Verification items for the finished model (mm, model axes). Face numbers are marked on the shaded views. A direction names the side the tool comes from. Give positions to 0.01 mm unless a question says otherwise; leave off trailing zeros. Write each loop counter-clockwise with the first axis right and the second up, starting at its lowest first coordinate (ties: lowest second). Pieces come first, ordered by that corner, then holes. Notation, with made-up numbers: (-0.5, 11.5) - (9.5, 11.5) arc R35 ccw to (9.5, 44.5) - close; hole circle Ø6 at (-22, 51). An arc over 180 degrees is marked (long way). Put each result on its own line as item: value.
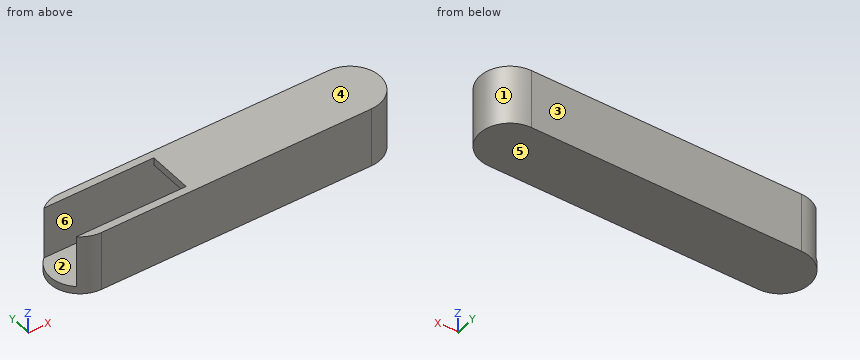
Autodesk Fusion 360 part; units mm, degrees
sketch "Sketch1" plane through (0, 0, 0) normal (0, 0, 1) x (1, 0, 0)
  line L0 (0, 0) -> (45, 0)
  line L1 (45, 10) -> (0, 10)
  arc A0 (0, 10) -> (0, 0) centre (0, 5) ccw
  arc A1 (45, 0) -> (45, 10) centre (45, 5) ccw
  dimension "d1" = 10
  dimension "d2" = 45
extrude "Extrude1" add sketch "Sketch1" along normal blind 10
sketch "Sketch2" plane through (0, 0, 0) normal (1, 0, 0) x (0, 1, 0)
  line L0 (1.25, 1.25) -> (8.75, 1.25)
  line L1 (8.75, 1.25) -> (8.75, 8.75)
  line L2 (8.75, 8.75) -> (1.25, 8.75)
  line L3 (1.25, 8.75) -> (1.25, 1.25)
  line L4 (10, 1.25) -> (8.75, 1.25) construction
  line L5 (0, 1.25) -> (1.25, 1.25) construction
  line L6 (0, 0) -> (0, 10)
  line L7 (10, 0) -> (10, 10)
  line L8 (8.75, 8.75) -> (8.75, 10) construction
  line L9 (8.75, 1.25) -> (8.75, 0) construction
  line L10 (10, 0) -> (0, 0)
  line L11 (10, 10) -> (0, 10)
  point P0 (10, 0)
  dimension "d5" = 7.5
  dimension "d6" = 7.5
extrude "Extrude2" cut sketch "Sketch2" along normal blind 45 and the other way through all contours L0 L1 L2 L3
sketch "Sketch3" plane through (0, 0, 10) normal (0, 0, 1) x (-1, 0, 0)
  arc A0 (-45, 0) -> (-45, -10) centre (-45, -5) ccw
  line L0 (-45, -10) -> (0, -10)
  arc A1 (0, -10) -> (0, 0) centre (0, -5) ccw
  line L1 (0, 0) -> (-45, 0)
  line L2 (5, -8.75) -> (-15, -8.75)
  line L3 (-15, -8.75) -> (-15, -1.25)
  line L4 (-15, -1.25) -> (5, -1.25)
  line L5 (5, -1.25) -> (5, -8.75)
  line L6 (5, -8.75) -> (5, -10) construction
  line L7 (5, -1.25) -> (5, 0) construction
  dimension "d11" = 7.5
  dimension "d12" = 30
extrude "Extrude3" cut sketch "Sketch3" against normal up to surface (1.25 mm away) contours A1 L2 L3 L4
Q1. Go/stop test with a flat-tipped pin: pin 1 Ø2 at (x, y) = (5.5, 4.5) entering from +Z. Record where the tip stops, or that it passes through.
Answers follow:
pin 1: stops at z = 1.25
Q2. Section check A-A, the plane x = 37.5. Record the cut outline in (y, z), plus the area to 4 significant figures.
Answers follow:
outline: (0, 0) - (10, 0) - (10, 10) - (0, 10) - close; hole (1.25, 1.25) - (8.75, 1.25) - (8.75, 8.75) - (1.25, 8.75) - close
area: 43.75 mm2
Q3. Section check C-C, the plane y = 5. Record the cut outline in (x, z), plus the area to 3 significant figures.
Answers follow:
outline: (-5, 0) - (50, 0) - (50, 10) - (15, 10) - (15, 8.75) - (45, 8.75) - (45, 1.25) - (-5, 1.25) - close
area: 150 mm2
Q4. Set-up check for the marked faces 5 and 6: record each of +Z, -Z, +X, -X, +Y, -Y from which the full face is reachable in a straight line by a thin tool's end or side.
Answers follow:
face 5: -Z, +X, -X, +Y, -Y
face 6: -X
Q5. Release check for a two-part mould opening along Y. For the marked faces 1, 2, 3 and 4 record: released by +Y, released by -Y, zero draft, split by the parting line, or undercut.
Answers follow:
face 1: split by the parting line
face 2: undercut
face 3: released by +Y
face 4: zero draft
Q6. Scan lines: line 1 along Y through (x, z) = (38.5, 1.75); line 2 along Z through (x, y) = (-0.5, 7.25). Record each from-to range of solid material in increasing order.
Answers follow:
line 1: y = 0 to 1.25, 8.75 to 10
line 2: z = 0 to 1.25
Q7. Section check B-B, the plane z = 1.75. Record the cut outline in (x, y), plus the area to 3 significant figures.
Answers follow:
outline: (-3.31, 1.25) arc R5 ccw to (0, 0) - (45, 0) arc R5 ccw to (45, 10) - (0, 10) arc R5 ccw to (-3.31, 8.75) - (45, 8.75) - (45, 1.25) - close
area: 157 mm2
